The listing builds one solid part. Answer for the finished solid, in the listing's coordinates (mm). Coordinates: 2 decimals unless noted, no trailing zeros. Loops run counter-clockwise (first coordinate to the right, second up) from the corner with the lowest first, then second, coordinate; pieces in that order, holes last. Notation, with made-up numbers: M 53.25,17 L 85.25,17 A23 ccw 85.25,53 Z; hole C 25.25,61.5 d8. An arc over 180 degrees is marked long. Answer as a JSON object with one key per item and string values. Group by question number.
1. A cutting plane is placed at D-D on y = -4. Give the vertices of the cut face in (x, z).
2. Straight lines are drawn through the part: L1, parallel to Y at x = 19, z = 0.7; L2, parallel to Y at x = -38.5, z = 2.65; L3, parallel to X at y = 25, z = 2. For each, find the intervals that lie inside material, in ascending order.
3. Determine the mould class of faces 1 (the face through (-10.696, 24.023, 1.479)), 2 (the face through (-35.455, 0.715, 1.479)), 3 (the face through (-13, -3, 0)) for opening direction Y: released by +Y, released by -Y, zero draft, split by the parting line, or undercut.
4. Given pin 1 (1 mm diameter, centred on x = -31.5, z = 2, fed in from -Y), flat-ended and moving along its own axis, determine where the tip first touches the part or whether it passes through.
5. A cutting plane is placed at A-A on y = -24.5. State how many separate pieces and enclosed holes the cut face has, and give its area (3 significant figures).
from build123d import *

# Parameters (mm, degrees)
SKETCH2_R           = 0.9
BOSS_EXTRUDE1_DEPTH = 3


with BuildPart() as part:
    # Sketch2 → Boss-Extrude1 (new body)
    with BuildSketch(Plane.XY):
        with BuildLine():
            add(Edge.make_bspline(
                [(-34.002851303, 8.604476718), (-58.333457607, 42.758566595), (-23.407809103, 21.030549249)],
                knots=[0, 0, 0, 1, 1, 1], degree=2))
            ThreePointArc((-34.002851303, 8.604476718), (-35.455837584, 0.600929894), (-34.105332305, -7.42054543))
            add(Edge.make_bspline(
                [(-34.105332305, -7.42054543), (-58.281676493, -42.050918016), (-23.642702616, -19.996916463)],
                knots=[0, 0, 0, 1, 1, 1], degree=2))
            ThreePointArc((-23.642702616, -19.996916463), (-11.029350737, -23.137049671), (1.333618717, -19.122816437))
            add(Edge.make_bspline(
                [(10.40030161, -7.407444616), (38.188248564, -42.452256001), (1.333618717, -19.122816437)],
                knots=[0, 0, 0, 1, 1, 1], degree=2))
            ThreePointArc((10.40030161, -7.407444616), (11.746657416, 0.460490628), (10.393307704, 8.32722588))
            add(Edge.make_bspline(
                [(10.393307704, 8.32722588), (38.116592963, 43.308207972), (1.359443986, 20.005390199)],
                knots=[0.00410137, 0.00410137, 0.00410137, 0.997962678, 0.997962678, 0.997962678], degree=2))
            ThreePointArc((1.359443986, 20.005390199), (-10.878759881, 24.031297997), (-23.407809103, 21.030549249))
        make_face()
        with Locations((-39, -24.5)):
            Circle(SKETCH2_R, mode=Mode.SUBTRACT)
        with Locations((19, -24.5)):
            Circle(SKETCH2_R, mode=Mode.SUBTRACT)
        with Locations((-39, 24.5)):
            Circle(SKETCH2_R, mode=Mode.SUBTRACT)
        with Locations((19, 24.5)):
            Circle(SKETCH2_R, mode=Mode.SUBTRACT)
    extrude(amount=BOSS_EXTRUDE1_DEPTH)


solid = part.part
From the geometry:
{
 "1": {"outline": "M -35.03,0 L 11.32,0 L 11.32,3 L -35.03,3 Z"},
 "2": {"L1": "y = -28.26 to -25.4, -23.6 to -19.2, 20.14 to 23.6, 25.4 to 29.14", "L2": "y = -27.93 to -25.25, -23.75 to -14.01, 15.22 to 23.75, 25.25 to 28.88", "L3": "x = -43.59 to -39.75, -38.25 to -30.13, 9.68 to 18.25, 19.75 to 21.64"},
 "3": {"face 1": "released by +Y", "face 2": "undercut", "face 3": "zero draft"},
 "4": {"pin 1": "stops at y = -24.96"},
 "5": {"separate pieces": "4", "enclosed holes": "0", "area": "61.4 mm²"}
}
